Autodesk Inventor part; units mm, degrees
ref_plane "YZ Plane" through (0, 0, 0) normal (1, 0, 0) x (0, 1, 0)
ref_plane "XZ Plane" through (0, 0, 0) normal (0, 1, 0) x (-1, 0, 0)
ref_plane "XY Plane" through (0, 0, 0) normal (0, 0, 1) x (1, 0, 0)
sketch "Sketch1" plane through (0, 0, 0) normal (0, 0, 1) x (1, 0, 0)
  line L0 (-384.81, 63.5) -> (384.81, 63.5)
  line L1 (384.81, 63.5) -> (384.81, -63.5)
  line L2 (384.81, -63.5) -> (-384.81, -63.5)
  line L3 (-384.81, -63.5) -> (-384.81, 63.5)
  point P0 (0, 0)
  point P1 (-384.81, 0)
  point P2 (0, 63.5)
  dimension "d0" = 769.62
  dimension "d1" = 127
extrude "Extrusion1" add sketch "Sketch1" along normal blind 19.05
sketch "Sketch2" plane through (0, 0, 0) normal (1, 0, 0) x (0, 1, 0)
  line L0 (63.5, 19.05) -> (63.5, 0) construction
  line L1 (63.5, 0) -> (-63.5, 0) construction
  line L2 (-63.5, 0) -> (-63.5, 19.05) construction
  line L3 (-63.5, 19.05) -> (63.5, 19.05) construction
  circle A0 centre (31.75, 50.8) radius 31.75
  circle A1 centre (-31.75, 50.8) radius 31.75
  point P0 (0, 0)
  dimension "d4" = 63.5
  dimension "d5" = 63.5
extrude "Extrusion2" add sketch "Sketch2" along normal mid plane 769.62
sketch "Sketch3" plane through (384.81, -63.5, 0) normal (1, 0, 0) x (0, 0, -1)
  line L0 (-19.05, 127) -> (0, 127)
  line L1 (0, 127) -> (0, 0)
  line L2 (0, 0) -> (-19.05, 0)
  line L3 (-19.05, 0) -> (-19.05, 31.75)
  line L4 (-19.05, 31.75) -> (-19.05, 95.25)
  arc A0 (-50.8, 63.5) -> (-19.05, 95.25) centre (-50.8, 95.25) ccw
  arc A1 (-50.8, 63.5) -> (-19.05, 31.75) centre (-50.8, 31.75) ccw
  arc A2 (-19.05, 31.75) -> (-50.8, 63.5) centre (-50.8, 31.75) ccw
  arc A3 (-19.05, 95.25) -> (-50.8, 63.5) centre (-50.8, 95.25) ccw
  line L5 (-19.05, 95.25) -> (-19.05, 127)
  line L6 (-50.8, 127) -> (-19.05, 127)
  line L7 (-82.55, 95.25) -> (-82.55, 31.75)
  line L8 (-50.8, 0) -> (-19.05, 0)
  point P0 (0, 63.5)
extrude "Extrusion3" add sketch "Sketch3" against normal blind 769.62 contours L5 A3 L6 | L4 A2 A0 | L3 L8 A1 | A1 L7 A3
fillet "Fillet1" radius 12.7 14 edges at (0, 63.5, 0) (384.81, 0, 0) (0, -63.5, 0) (-384.81, 0, 0) (-384.81, 63.5, 25.4) (384.81, 63.5, 25.4) (-384.81, 54.2006, 73.2506) (-384.81, 0, 82.55) (-384.81, -54.2006, 73.2506) (-384.81, -63.5, 25.4) (384.81, 54.2006, 73.2506) (384.81, 0, 82.55) (384.81, -54.2006, 73.2506) (384.81, -63.5, 25.4)
equation "\"d6\" = d0"
equation "\"d8\" = d0"
properties part number "FrontBumpers"
Here's how the part is built. I have some questions about the finished solid (model axes, mm). Round coordinates to 2 decimals unless told otherwise and drop trailing zeros. Order: outer loops, then holes, each group sorted by start corner. A loop starts at its lowest first (then second) coordinate and runs counter-clockwise, first axis right, second up. Notation, with made-up numbers: M 14,41 L 52,41 A24 cw 52,66 Z; hole C 73,71 d6. An arc over 180 degrees is marked long. Answer in a Markdown table with one row per item.
Item 1: If I drill on L1, parallel to Y at x = -100, z = 51; L2, parallel to Z at x = 9, y = -32; L3, parallel to X at y = -50.5, z = 62, over which ranges is the centre line in solid material (lowest first)? Write a range as from..to.
A:
| item | result |
|---|---|
| L1 | y = -63.5..63.5 |
| L2 | z = 0..82.55 |
| L3 | x = -384.5..384.5 |
Item 2: I'm going to push flat-ended pins straight in: pin 1 (2 mm diameter, centred on x = -141.5, y = 45, fed in from +Z); pin 2 (8 mm diameter, centred on x = 255, z = 72.5, fed in from +Y); pin 3 (8 mm diameter, centred on x = -5.5, y = -9.5, fed in from -Z). Where does each tip first touch, or does it pass through?
A:
| item | result |
|---|---|
| pin 1 | stops at z = 80.09 |
| pin 2 | stops at y = 58.11 |
| pin 3 | stops at z = 0 |
Item 3: Imagine slicing it at A-A, the plane x = 257. Write out the boundary of the cut face in (y, z), and give its area (3 significant figures).
A:
| item | result |
|---|---|
| outline | M -63.5,12.7 A12.7 ccw -50.8,0 L 50.8,0 A12.7 ccw 63.5,12.7 L 63.5,50.8 A31.75 ccw 31.75,82.55 L -31.75,82.55 A31.75 ccw -63.5,50.8 Z |
| area | 9,980 mm2 |
Item 4: Thinking about a two-plate mould opening in Y: for faces 1 (the face through (-380.99, -59.88, 31.48)), 2 (the face through (-5.21, 53.95, 73.5)), 3 (the face through (-5, 1, 0)), which applies, +Y half, -Y half, draft (parallel to the pull), parting line (faces both ways), or undercut?
A:
| item | result |
|---|---|
| face 1 | -Y half |
| face 2 | +Y half |
| face 3 | draft |
